```python
from build123d import *

# Parameters (mm, degrees)
BOSS_EXTRUSION_DEPTH     = 5.5
SCHIZZO2_W               = 7.7
SCHIZZO2_H               = 15
EXTERNAL_EXTRUSION_DEPTH = 13.5
SCHIZZO3_R               = 1.9
CETRAL_HOLE_DEPTH        = 6.5
SKETCH1_R                = 1.5
CUT_EXTRUDE1_DEPTH       = 7.7
CIRPATTERN1_COUNT        = 3
FILLET1_R                = 10
FILLET2_R                = 4
FILLET3_R                = 2
SKETCH2_R                = 0.5
CUT_EXTRUDE2_DEPTH       = 7.7
SKETCH2_5_W              = 1
SKETCH2_5_H              = 8
SKETCH2_5_W_2            = 10
SKETCH2_5_H_2            = 1
BOSS_EXTRUDE1_DEPTH      = 7.5
FILLET4_R                = 2
CHAMFER1_SIZE            = 2
SKETCH2_6_R              = 1.2
SKETCH2_6_R_2            = 1.9
SKETCH2_6_R_3            = 0.5
CUT_EXTRUDE4_DEPTH       = 1.5
CUT_EXTRUDE5_START       = -5.5
SKETCH2_7_R              = 1.2
SKETCH2_7_R_2            = 0.5
CUT_EXTRUDE5_DEPTH       = 1.5
SKETCH4_R                = 2.5
CUT_EXTRUDE6_DEPTH       = 0.7


with BuildPart() as part:
    # Schizzo1 → Boss extrusion (new body)
    with BuildSketch(Plane(origin=(0, 0, 0), x_dir=(1, 0, 0), z_dir=(0, 1, 0))):
        Polygon((-27.611313476, 11.495802195), (-14.620932419, 3.995802195), (-14.620932419, -8.441399268), (-3.85, -14.66), (-3.85, -29.66), (3.85, -29.66), (3.85, -14.66), (14.620932419, -8.441399268), (14.620932419, 3.995802195), (27.611313476, 11.495802195), (23.761313476, 18.164197805), (10.770932419, 10.664197805), (0, 16.882798536), (-10.770932419, 10.664197805), (-23.761313476, 18.164197805), align=None)
    extrude(amount=BOSS_EXTRUSION_DEPTH)

    # Schizzo2 → external extrusion (add)
    with BuildSketch(Plane(origin=(0, 5.5, 0), x_dir=(1, 0, 0), z_dir=(0, 1, 0))):
        Polygon((-23.761313476, 18.164197805), (-27.611313476, 11.495802195), (-14.620932419, 3.995802195), (-10.770932419, 10.664197805), align=None)
        with Locations((0, -22.16)):
            Rectangle(SCHIZZO2_W, SCHIZZO2_H)
        Polygon((10.770932419, 10.664197805), (14.620932419, 3.995802195), (27.611313476, 11.495802195), (23.761313476, 18.164197805), align=None)
    extrude(amount=EXTERNAL_EXTRUSION_DEPTH)

    # Schizzo3 → cetral hole (cut, through all)
    with BuildSketch(Plane(origin=(0, 5.5, 0), x_dir=(1, 0, 0), z_dir=(0, 1, 0))):
        Circle(SCHIZZO3_R)
    extrude(amount=-CETRAL_HOLE_DEPTH, mode=Mode.SUBTRACT)

    # Sketch1 → Cut-Extrude1 (cut)
    with BuildSketch(Plane.ZY.offset(3.85)):
        with Locations((17.66, 15.5)):
            Circle(SKETCH1_R)
        with Locations((25.41, 15.5)):
            Circle(SKETCH1_R)
        Polygon((29.66, 19), (29.66, 0), (25.66, 0), align=None)
    cut_extrude1 = extrude(amount=-CUT_EXTRUDE1_DEPTH, mode=Mode.SUBTRACT)

    # CirPattern1: Cut-Extrude1 ×3 about axis
    cirpattern1_axis = Axis((0, 0, 0), (0, 1, 0))
    for i in range(1, CIRPATTERN1_COUNT):
        add(cut_extrude1.rotate(cirpattern1_axis, i * 360 / CIRPATTERN1_COUNT), mode=Mode.SUBTRACT)

    # Fillet1
    fillet1_edges = [part.edges().sort_by_distance(p)[0] for p in [
        (-3.85, 2.75, 14.66),
        (-14.620932419, 2.75, 8.441399268),
        (-14.620932419, 2.75, -3.995802195),
        (-10.770932419, 2.75, -10.664197805),
        (0, 2.75, -16.882798536),
        (10.770932419, 2.75, -10.664197805),
        (14.620932419, 2.75, -3.995802195),
        (14.620932419, 2.75, 8.441399268),
        (3.85, 2.75, 14.66),
    ]]
    fillet(fillet1_edges, radius=FILLET1_R)

    # Fillet2
    fillet2_edges = [part.edges().sort_by_distance(p)[0] for p in [
        (-12.695932419, 19, -7.33),
        (0, 19, 14.66),
        (12.695932419, 19, -7.33),
    ]]
    fillet(fillet2_edges, radius=FILLET2_R)

    # Fillet3
    fillet3_edges = [part.edges().sort_by_distance(p)[0] for p in [
        (-25.686313476, 19, -14.83),
        (0, 19, 29.66),
        (25.686313476, 19, -14.83),
    ]]
    fillet(fillet3_edges, radius=FILLET3_R)

    # Sketch2 → Cut-Extrude2 (cut)
    with BuildSketch(Plane.XZ):
        with Locations((-4.5, 0)):
            Circle(SKETCH2_R)
        with Locations((4.5, 0)):
            Circle(SKETCH2_R)
    extrude(amount=-CUT_EXTRUDE2_DEPTH, mode=Mode.SUBTRACT)

    # Sketch2<5> → Boss-Extrude1 (add)
    with BuildSketch(Plane.XZ):
        with Locations((6.5, 0)):
            Rectangle(SKETCH2_5_W, SKETCH2_5_H)
        with Locations((0, 5.5)):
            Rectangle(SKETCH2_5_W_2, SKETCH2_5_H_2)
        with Locations((-6.5, 0)):
            Rectangle(SKETCH2_5_W, SKETCH2_5_H)
        with Locations((0, -5.5)):
            Rectangle(SKETCH2_5_W_2, SKETCH2_5_H_2)
    extrude(amount=BOSS_EXTRUDE1_DEPTH)

    # Fillet4
    fillet4_edges = [part.edges().sort_by_distance(p)[0] for p in [
        (6.5, -7.5, 4),
        (6.5, -7.5, -4),
        (-5, -7.5, 5.5),
        (5, -7.5, 5.5),
        (-6.5, -7.5, -4),
        (-6.5, -7.5, 4),
        (5, -7.5, -5.5),
        (-5, -7.5, -5.5),
    ]]
    fillet(fillet4_edges, radius=FILLET4_R)

    # Chamfer1
    chamfer1_edges = [part.edges().sort_by_distance(p)[0] for p in [
        (7, 0, 0),
        (0, 0, 6),
        (-7, 0, 0),
        (0, 0, -6),
    ]]
    chamfer(chamfer1_edges, length=CHAMFER1_SIZE)

    # Sketch2<6> → Cut-Extrude4 (cut)
    with BuildSketch(Plane.XZ):
        Polygon((-6, 4), (-6, -4), (-6, -5), (-5, -5), (5, -5), (6, -5), (6, -4), (6, 4), (6, 5), (5, 5), (-5, 5), (-6, 5), align=None)
        with Locations((-4.5, 0)):
            Circle(SKETCH2_6_R, mode=Mode.SUBTRACT)
        Circle(SKETCH2_6_R_2, mode=Mode.SUBTRACT)
        with Locations((4.5, 0)):
            Circle(SKETCH2_6_R, mode=Mode.SUBTRACT)
        with Locations((-4.5, 0)):
            Circle(SKETCH2_6_R)
        with Locations((-4.5, 0)):
            Circle(SKETCH2_6_R_3, mode=Mode.SUBTRACT)
        with Locations((4.5, 0)):
            Circle(SKETCH2_6_R)
        with Locations((4.5, 0)):
            Circle(SKETCH2_6_R_3, mode=Mode.SUBTRACT)
    extrude(amount=-CUT_EXTRUDE4_DEPTH, mode=Mode.SUBTRACT)

    # Sketch2<7> → Cut-Extrude5 (cut)
    with BuildSketch(Plane.XZ.offset(CUT_EXTRUDE5_START)):
        with Locations((-4.5, 0)):
            Circle(SKETCH2_7_R)
        with Locations((-4.5, 0)):
            Circle(SKETCH2_7_R_2, mode=Mode.SUBTRACT)
        with Locations((4.5, 0)):
            Circle(SKETCH2_7_R)
        with Locations((4.5, 0)):
            Circle(SKETCH2_7_R_2, mode=Mode.SUBTRACT)
    extrude(amount=CUT_EXTRUDE5_DEPTH, mode=Mode.SUBTRACT)

    # Sketch4 → Cut-Extrude6 (cut)
    with BuildSketch(Plane.XZ.offset(-1.5)):
        Circle(SKETCH4_R)
    extrude(amount=-CUT_EXTRUDE6_DEPTH, mode=Mode.SUBTRACT)


solid = part.part
```
The listing builds one solid part. Answer for the finished solid, in the listing's coordinates (mm). A direction names the side the tool comes from. Coordinates: 2 decimals unless noted, no trailing zeros. Write each loop counter-clockwise with the first axis right and the second up, starting at its lowest first coordinate (ties: lowest second). Pieces come first, ordered by that corner, then holes. Notation, with made-up numbers: (62, -1.5) - (69, -1.5) arc R38 cw to (69, 36.5) - close; hole circle Ø3 at (77.5, 43). An arc over 180 degrees is marked (long way). Return JSON: item names as keys, results as strings. Group by question number.
Q1. For a pull along X with two mould halves and no side action, classify faces 1 (the flat face through (0, 10, 14.66)), 2 (the flat face through (-5, -2.1, -5.85)), 3 (the cylindrical face through (-0.54, 1.85, -2.44)) as +X half, -X half, draft (parallel to the pull), parting line (faces both ways), or undercut.
Q2. The part is cut by section B-B on y = 11. Write down the section's boundary in (x, z).
Q3. The part is cut by section A-A on y = -3.75. Write down the section's boundary in (x, z), and give its area (3 significant figures).
Q4. Find the intervals of material crossed by line 1 along Y through (x, z) = (7, 11.5); line 2 along Z through (x, y) = (0, 2.05); line 3 along Y through (x, z) = (0, 25), in increasing order. Write a range as [from, to].
Q5. The part is cut by section C-C on z = 17.66. Write down the section's boundary in (x, y), and give its area (3 significant figures).
Q6. Flat-ended cylindrical pins translate along their axes: pin 1 Ø3 at (x, y) = (0, -4.5) entering from -Z; pin 2 Ø1 at (y, z) = (4, 2.5) entering from -X; pin 3 Ø10 at (y, z) = (-3.5, 1.5) entering from -X; pin 4 Ø2.5 at (y, z) = (15.5, 17.66) entering from -X. Find the tip coordinate at first contact, or state that the pin passes through.
Q7. The part is cut by section D-D on z = 9.5. Write down the section's boundary in (x, y).
Q8. Which of the six approach directions +Z, -Z, +X, -X, +Y, -Y give full straight-line access (tool end or side, diameter ignored) to faces 4 (the flat face through (5, -2.1, 5.8)), 5 (the flat face through (3.85, 11, 22)), 6 (the flat face through (12.669, 10.183, -7.377)), 7 (the flat face through (-6.85, -2.1, -4)), 8 (the flat face through (0, -5, 6))?
Evaluation:
{
 "1": {"face 1": "draft", "face 2": "-X half", "face 3": "undercut"},
 "2": {"outline": "(-26.15, -10.65) - (-22.3, -17.32) - (-10.77, -10.66) - (-14.62, -4) - close; (-3.85, 14.66) - (3.85, 14.66) - (3.85, 27.98) - (-3.85, 27.98) - close; (10.77, -10.66) - (22.3, -17.32) - (26.15, -10.65) - (14.62, -4) - close"},
 "3": {"outline": "(-7, -4) - (-6, -4) - (-6, 4) - (-7, 4) - close; (-5, -6) - (5, -6) - (5, -5) - (-5, -5) - close; (-5, 5) - (5, 5) - (5, 6) - (-5, 6) - close; (6, -4) - (7, -4) - (7, 4) - (6, 4) - close", "area": "36.0 mm2"},
 "4": {"line 1": "y = [0, 5.5]", "line 2": "z = [-15.34, -2.5], [2.5, 26.09]", "line 3": "y = [0, 14.06], [16.94, 19]"},
 "5": {"outline": "(-4.24, 0) - (4.24, 0) - (4.24, 5.5) - (3.85, 5.5) - (3.85, 14) - (-3.85, 14) - (-3.85, 5.5) - (-4.24, 5.5) - close; (-3.85, 17) - (3.85, 17) - (3.85, 18.87) - (-3.85, 18.87) - close", "area": "127 mm2"},
 "6": {"pin 1": "stops at z = -6", "pin 2": "stops at x = -14.62", "pin 3": "stops at x = -15.39", "pin 4": "passes through"},
 "7": {"outline": "(-11.92, 0) - (11.92, 0) - (11.92, 5.5) - (-11.92, 5.5) - close"},
 "8": {"face 4": "+Z, -Z, +X, -Y", "face 5": "+Z, +X, +Y", "face 6": "+Z, +Y", "face 7": "-Z, +X, -X, -Y", "face 8": "+Z, +X, -X, -Y"}
}
